The figure shows three views and two pictorial views of one solid part (mm, origin at its lowest corner). Answer the questions. Coordinates: 2 decimals unless noted, no trailing zeros. Order: outer loops, then holes, each group sorted by start corner. A loop starts at its lowest first (then second) coordinate and runs counter-clockwise, first axis right, second up. Notation, with made-up numbers: (45, 12) -> (49, 12) arc R34 ccw to (49, 42) -> close; hole circle Ø1 at (56, 45.5). An arc over 180 degrees is marked (long way). Return JSON: item names as keys, results as strings.
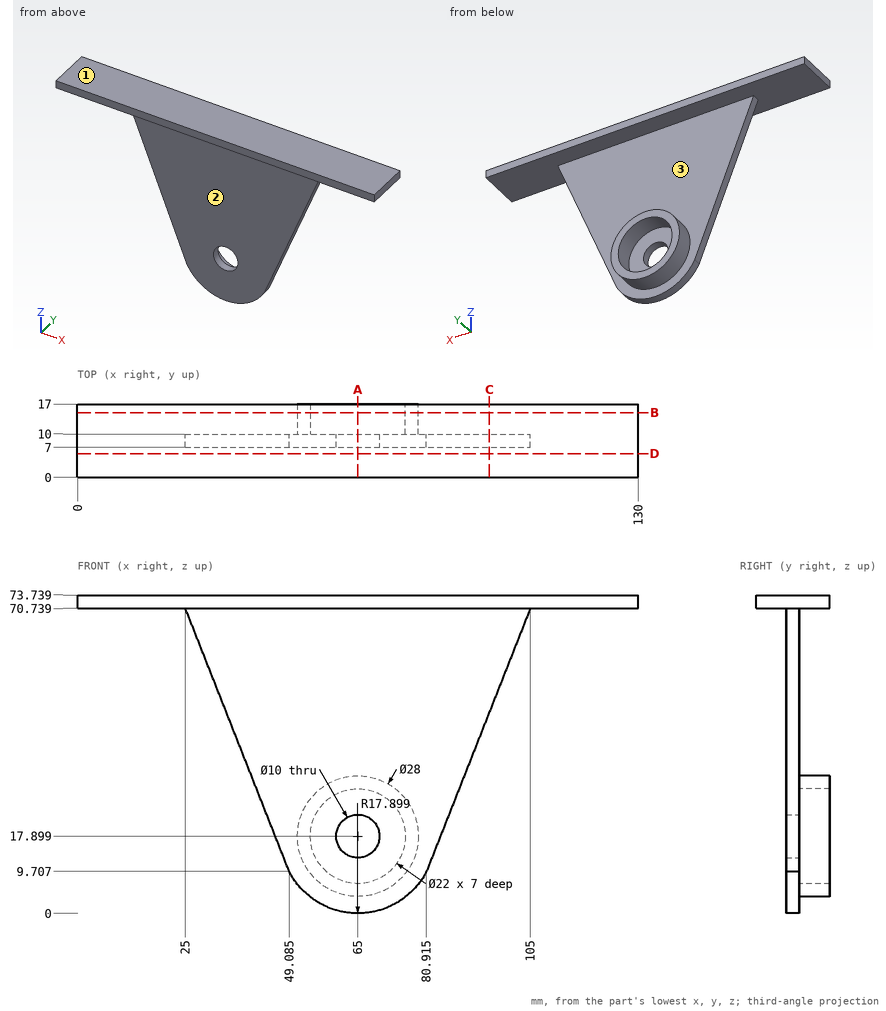
1. Consider line 1 (Z direction, x = 65, y = 11.5); line 2 (Z direction, x = 57.5, y = 15.5) (1 decimal); line 3 (Y direction, x = 58.5, z = 67). Determine where each line is inside the solid, lowest interval first. Write a range as from..to.
Answer block:
{"line 1": "z = 3.9..6.9, 28.9..31.9, 70.74..73.74", "line 2": "z = 6.1..9.9, 25.9..29.7, 70.7..73.7", "line 3": "y = 7..10"}
2. The part is cut by section D-D on y = 5.5. Give the vertices of the cut face in (x, z).
Answer block:
{"outline": "(0, 70.74) -> (130, 70.74) -> (130, 73.74) -> (0, 73.74) -> close"}
3. The part is cut by section A-A on x = 65. Give the vertices of the cut face in (y, z), and give its area (3 significant figures).
Answer block:
{"outline": "(0, 70.74) -> (7, 70.74) -> (7, 22.9) -> (10, 22.9) -> (10, 28.9) -> (17, 28.9) -> (17, 31.9) -> (10, 31.9) -> (10, 70.74) -> (17, 70.74) -> (17, 73.74) -> (0, 73.74) -> close; (7, 0) -> (10, 0) -> (10, 3.9) -> (17, 3.9) -> (17, 6.9) -> (10, 6.9) -> (10, 12.9) -> (7, 12.9) -> close", "area": "275 mm2"}
4. The part is cut by section C-C on x = 95.5. Give the vertices of the cut face in (y, z).
Answer block:
{"outline": "(0, 70.74) -> (7, 70.74) -> (7, 46.67) -> (10, 46.67) -> (10, 70.74) -> (17, 70.74) -> (17, 73.74) -> (0, 73.74) -> close"}
5. Each of these flat-tipped pins is pushed along its axis until it touches: pin 1 Ø1.5 at (y, z) = (8.5, 16) entering from +X; pin 2 Ø1 at (x, z) = (81.5, 32.5) entering from +Y; pin 3 Ø4 at (y, z) = (9, 21.5) entering from +X. Where does it stop, or does it pass through?
Answer block:
{"pin 1": "stops at x = 83.69", "pin 2": "stops at y = 10", "pin 3": "stops at x = 86.36"}
6. The part is cut by section B-B on y = 15. Give the vertices of the cut face in (x, z).
Answer block:
{"outline": "(0, 70.74) -> (130, 70.74) -> (130, 73.74) -> (0, 73.74) -> close; circle Ø28 at (65, 17.9); hole circle Ø22 at (65, 17.9)"}
7. Determine the mould class of the marked faces 1, 2 and 3 for opening direction Z: pulls with the +Z half, pulls with the -Z half, needs draft (parallel to the pull), parting line crosses it, or undercut.
Answer block:
{"face 1": "pulls with the +Z half", "face 2": "needs draft", "face 3": "undercut"}
